Here's how the part is built. I have some questions about the finished solid (model axes, mm). Coordinates: 2 decimals unless noted, no trailing zeros. Order: outer loops, then holes, each group sorted by start corner. A loop starts at its lowest first (then second) coordinate and runs counter-clockwise, first axis right, second up. Notation, with made-up numbers: (68.25, 51) - (115.25, 51) arc R18 cw to (115.25, 56) - close; hole circle Ø10 at (84.5, -2). An arc over 180 degrees is marked (long way). Answer in a Markdown table with one row per item. Add a question column.
Item 1: If I drill on line 1 along X through (y, z) = (0.5, -7.5); line 2 along X through (y, z) = (1.1, -7.75); line 3 along X through (y, z) = (1.6, -5.5), over which ranges is the centre line in solid material (lowest first)? Write a range as from..to.
Item 2: I want a section at C-C (y = 0.8). Count the separate pieces of the cut face and the enclosed holes in it, plus the area to 3 significant figures.
Item 3: I want a section at A-A (z = -6). Please give me the cut outline in (x, y), plus the area to 3 significant figures.
Item 4: I want a section at B-B (x = 10.5). Please give me the cut outline in (y, z), plus the area to 3 significant figures.
Item 5: Thinking about a two-plate mould opening in Z: for faces 1 (the cylindrical face through (-16.99, 0.99, -7.16)), 2 (the cylindrical face through (11.102, 0.986, -5.386)), 3 (the cylindrical face through (12.638, 0.986, -7.826)), which applies, +Z half, -Z half, draft (parallel to the pull), parting line (faces both ways), or undercut?
```python
from build123d import *

# Parameters (mm, degrees)
SKETCH2_R           = 2.000000006
BOSS_EXTRUDE1_DEPTH = 2


with BuildPart() as part:
    # Sketch2 → Boss-Extrude1 (new body)
    with BuildSketch(Plane(origin=(0, 0, 0), x_dir=(1, 0, 0), z_dir=(0, 1, 0))):
        with BuildLine():
            ThreePointArc((-27.926975425, 9.714102761), (-29.649166118, 4.682637411), (-24.412176183, 3.757693749))
            ThreePointArc((-24.412176183, 3.757693749), (-16.874008703, 7.178664325), (-8.63567196, 6.368222256))
            ThreePointArc((-8.63567196, 6.368222256), (0.414236301, 2.94154028), (10.090788082, 3.027182087))
            ThreePointArc((10.090788082, 3.027182087), (12.602603797, 7.907109409), (7.276457736, 9.231902599))
            add(Edge.make_bspline(
                [(7.276457736, 9.231902599), (4.991666248, 8.239417516), (-0.384919766, 8.392254408), (-11.300329238, 15.23385505), (-22.195691788, 12.013740113), (-27.926975425, 9.714102761)],
                knots=[0.02947385, 0.02947385, 0.02947385, 0.02947385, 0.205279709, 0.474213823, 1, 1, 1, 1], degree=3))
        make_face()
        with Locations(Location((-26.634838433, 6.461352848, 0), (0, 0, 270))):
            Circle(SKETCH2_R, mode=Mode.SUBTRACT)
        with Locations(Location((9.415161567, 6.461352848, 0), (0, 0, 270))):
            Circle(SKETCH2_R, mode=Mode.SUBTRACT)
    extrude(amount=BOSS_EXTRUDE1_DEPTH)


solid = part.part
```
Values follow:
| question | item | result |
|---|---|---|
| 1 | line 1 | x = -29.98..-28.34, -24.93..7.71, 11.12..12.76 |
| 1 | line 2 | x = -29.89..-28.16, -25.11..7.89, 10.94..12.67 |
| 1 | line 3 | x = -30..-28.39, -24.88..-21.81, -7.1..7.66, 11.17..12.78 |
| 2 | separate pieces | 1 |
| 2 | enclosed holes | 2 |
| 2 | area | 238 mm^2 |
| 3 | outline | (-30.1, 0) - (-28.58, 0) - (-28.58, 2) - (-30.1, 2) - close; (-24.69, 0) - (-20.79, 0) - (-20.79, 2) - (-24.69, 2) - close; (-8.01, 0) - (7.47, 0) - (7.47, 2) - (-8.01, 2) - close; (11.36, 0) - (12.88, 0) - (12.88, 2) - (11.36, 2) - close |
| 3 | area | 44.9 mm^2 |
| 4 | outline | (0, -9.79) - (2, -9.79) - (2, -8.14) - (0, -8.14) - close; (0, -4.78) - (2, -4.78) - (2, -3.13) - (0, -3.13) - close |
| 4 | area | 6.59 mm^2 |
| 5 | face 1 | +Z half |
| 5 | face 2 | undercut |
| 5 | face 3 | parting line |
